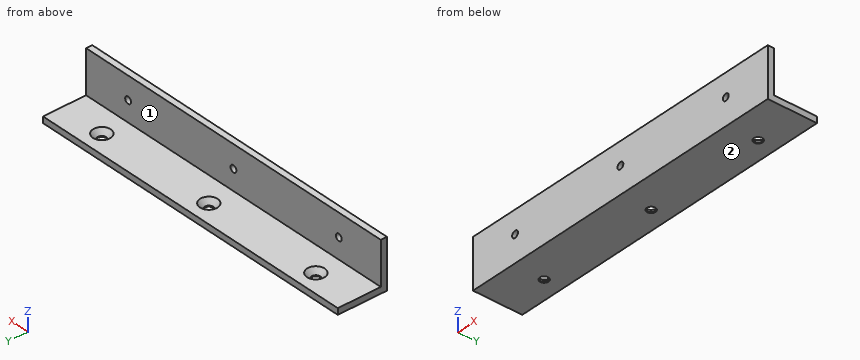
```python
from build123d import *

# Parameters (mm, degrees)
SKETCH1_W                                     = 174.879
SKETCH1_H                                     = 25.4
BOSS_EXTRUDE1_DEPTH                           = 3.175
SKETCH2_W                                     = 174.879
SKETCH2_H                                     = 3.175
BOSS_EXTRUDE2_DEPTH                           = 22.225
F_8_32_TAPPED_HOLE1_D                         = 3.4544
F_8_32_TAPPED_HOLE1_DEPTH                     = 10.668
F_8_32_TAPPED_HOLE1_TIP                       = 1.037806461
CSK_FOR_8_FLAT_HEAD_SOCKET_CAP_SCREW1_A_COUNT = 2
CSK_FOR_8_FLAT_HEAD_SOCKET_CAP_SCREW1_A_PITCH = 63.5
CSK_FOR_8_FLAT_HEAD_SOCKET_CAP_SCRE_2_COUNT   = 2
CSK_FOR_8_FLAT_HEAD_SOCKET_CAP_SCRE_2_PITCH   = 127


with BuildPart() as part:
    # Sketch1 → Boss-Extrude1 (new body)
    with BuildSketch(Plane(origin=(0, 0, 0), x_dir=(1, 0, 0), z_dir=(0, 1, 0))):
        Rectangle(SKETCH1_W, SKETCH1_H)
    extrude(amount=BOSS_EXTRUDE1_DEPTH)

    # Sketch2 → Boss-Extrude2 (add)
    with BuildSketch(Plane(origin=(0, 3.175, 0), x_dir=(1, 0, 0), z_dir=(0, 1, 0))):
        with Locations((0, 11.1125)):
            Rectangle(SKETCH2_W, SKETCH2_H)
    extrude(amount=BOSS_EXTRUDE2_DEPTH)

    # #8-32 Tapped Hole1
    with Locations(Plane(origin=(0, 3.175, 0), x_dir=(-1, 0, 0), z_dir=(0, 1, 0))):
        with Locations((62.5, 1.016), (0, 1.016), (-62.5, 1.016)):
            Hole(F_8_32_TAPPED_HOLE1_D / 2, depth=F_8_32_TAPPED_HOLE1_DEPTH)
            with Locations((0, 0, -(F_8_32_TAPPED_HOLE1_DEPTH + F_8_32_TAPPED_HOLE1_TIP / 2))):  # 118° drill point
                Cone(0, F_8_32_TAPPED_HOLE1_D / 2, F_8_32_TAPPED_HOLE1_TIP, mode=Mode.SUBTRACT)

    # Sketch6 → CSK for #8 Flat Head Socket Cap Screw1 (revolve, cut)
    with BuildSketch(Plane(origin=(-63.5, 15.875, -9.525), x_dir=(0, -1, 0), z_dir=(1, 0, 0))):
        Polygon((0, 0), (0, 3.175), (2.2479, 3.175), (2.2479, 2.658961536), (4.5593, 0), align=None)
    csk_for_8_flat_head_socket_cap_screw1 = revolve(axis=Axis((-63.5, 15.875, -3.175), (0, 0, -1)), mode=Mode.SUBTRACT)

    # CSK for #8 Flat Head Socket Cap Screw1 a: CSK for #8 Flat Head Socket Cap Screw1 ×2
    with Locations(*[(i * CSK_FOR_8_FLAT_HEAD_SOCKET_CAP_SCREW1_A_PITCH, 0, 0) for i in range(1, CSK_FOR_8_FLAT_HEAD_SOCKET_CAP_SCREW1_A_COUNT)]):
        add(csk_for_8_flat_head_socket_cap_screw1, mode=Mode.SUBTRACT)

    # CSK for _8 Flat Head Socket Cap Scre 2: CSK for #8 Flat Head Socket Cap Screw1 ×2
    with Locations(*[(i * CSK_FOR_8_FLAT_HEAD_SOCKET_CAP_SCRE_2_PITCH, 0, 0) for i in range(1, CSK_FOR_8_FLAT_HEAD_SOCKET_CAP_SCRE_2_COUNT)]):
        add(csk_for_8_flat_head_socket_cap_screw1, mode=Mode.SUBTRACT)


solid = part.part
```
Input: part model. Units: mm. Frame: model coordinates. Face numbers are marked on the shaded views. A direction names the side the tool comes from. Give positions to 0.01 mm unless a question says otherwise; leave off trailing zeros. Order: outer loops, then holes, each group sorted by start corner. A loop starts at its lowest first (then second) coordinate and runs counter-clockwise, first axis right, second up. Notation, with made-up numbers: M 72.5,-11 L 120.5,-11 A33 ccw 120.5,17 Z; hole C -3.75,65.25 d5. An arc over 180 degrees is marked long. Return JSON: item names as keys, results as strings.
1) Section query B-B on z = 5.5. Output: boundary loops of the cut face in (x, y) (1 decimal), and give its area (3 significant figures).
Taken from the geometry:
{"outline": "M -87.4,0 L 87.4,0 L 87.4,3.2 L -87.4,3.2 Z", "area": "555 mm2"}
2) Contact query for flat-ended pins moving along their axis: pin 1 (5.5 mm diameter, centred on x = -62.5, z = 1.016, fed in from +Y) (3 decimals); pin 2 (3 mm diameter, centred on x = -1.5, y = 15.5, fed in from +Z); pin 3 (3 mm diameter, centred on x = 0, z = 1.016, fed in from -Y); pin 4 (11 mm diameter, centred on x = 13.5, y = 12, fed in from +Z) (3 decimals). Output: stop coordinate, or through.
Taken from the geometry:
{"pin 1": "stops at y = 3.175", "pin 2": "stops at z = -11.27", "pin 3": "passes through", "pin 4": "stops at z = -9.525"}
3) Access query for the marked faces 1 and 2. Directions: +Z, -Z, +X, -X, +Y, -Y. A direction counts if a zero-diameter tool reaches every point of the face in a straight line with its end or side. Return the directions, or none.
Taken from the geometry:
{"face 1": "+Z, +X, -X, +Y", "face 2": "-Z, +X, -X, +Y, -Y"}
4) Section query D-D on y = 5.75. Output: boundary loops of the cut face in (x, z) (1 decimal).
Taken from the geometry:
{"outline": "M -87.4,-12.7 L 87.4,-12.7 L 87.4,-9.5 L -87.4,-9.5 Z"}
5) Line query: L1, parallel to Y at x = -63.5, z = -12.55; L2, parallel to Z at x = 0, y = 1.95; L3, parallel to Y at x = 62.5, z = -6.25 (3 decimals). Output: solid intervals per line, ascending. Write a range as [from, to].
Taken from the geometry:
{"L1": "y = [0, 13.63], [18.12, 25.4]", "L2": "z = [-12.7, -0.71], [2.74, 12.7]", "L3": "y = [0, 3.175]"}
6) Section query A-A on x = 0. Output: boundary loops of the cut face in (y, z) (3 decimals), and give its area (3 significant figures).
Taken from the geometry:
{"outline": "M 0,-12.7 L 13.627,-12.7 L 13.627,-12.184 L 11.316,-9.525 L 3.175,-9.525 L 3.175,-0.711 L 0,-0.711 Z; M 0,2.743 L 3.175,2.743 L 3.175,12.7 L 0,12.7 Z; M 18.123,-12.7 L 25.4,-12.7 L 25.4,-9.525 L 20.434,-9.525 L 18.123,-12.184 Z", "area": "120 mm2"}
7) Section query C-C on x = 51. Output: boundary loops of the cut face in (y, z) (3 decimals).
Taken from the geometry:
{"outline": "M 0,-12.7 L 25.4,-12.7 L 25.4,-9.525 L 3.175,-9.525 L 3.175,12.7 L 0,12.7 Z"}
